from build123d import *

# Parameters (mm, degrees)
BOSS_EXTRUDE1_DEPTH      = 25
CUT_EXTRUDE1_DEPTH       = 4
FILLET1_R                = 4
FILLET2_R                = 10
FILLET3_R                = 5
FILLET4_R                = 3
BOSS_EXTRUDE2_DEPTH      = 3
BOSS_EXTRUDE2_DEPTH_BACK = 3
FILLET5_R                = 3


with BuildPart() as part:
    # Sketch1 → Boss-Extrude1 (new body)
    with BuildSketch(Plane(origin=(0, 0, 0), x_dir=(0, 0, -1), z_dir=(1, 0, 0))):
        Polygon((0, 0), (-130, 0), (-130, 5), (-100.000366453, 5.148280317), (-77.868517379, 27.5), (101.088229162, 27.5), (114, 18), (114, 0), (74, 0), (74, 7.5), (0, 7.5), align=None)
    extrude(amount=BOSS_EXTRUDE1_DEPTH)

    # Sketch4 → Cut-Extrude1 (cut)
    with BuildSketch(Plane(origin=(25, 0, 0), x_dir=(0, 0, -1), z_dir=(1, 0, 0))):
        Polygon((-100.876178749, 0), (0, 0), (111, 0), (111, 3), (111, 16.482758557), (100.103496394, 24.5), (-76.617181678, 24.5), align=None)
    cut_extrude1 = extrude(amount=-CUT_EXTRUDE1_DEPTH, mode=Mode.SUBTRACT)

    # Mirror2: Cut-Extrude1 across plane
    add(cut_extrude1.mirror(Plane(origin=(12.5, 0, 0), x_dir=(0, 0, 1), z_dir=(1, 0, 0))), mode=Mode.SUBTRACT)

    # Fillet1
    fillet1_edges = [part.edges().sort_by_distance(p)[0] for p in [
        (12.5, 7.5, -74),
        (12.5, 7.5, 0),
    ]]
    fillet(fillet1_edges, radius=FILLET1_R)

    # Fillet2
    fillet2_edges = [part.edges().sort_by_distance(p)[0] for p in [
        (23, 0, 100.876178749),
        (23, 24.5, 76.617181678),
        (23, 24.5, -100.103496394),
        (23, 16.482758557, -111),
        (2, 0, 100.876178749),
        (2, 16.482758557, -111),
        (2, 24.5, -100.103496394),
        (2, 24.5, 76.617181678),
    ]]
    fillet(fillet2_edges, radius=FILLET2_R)

    # Fillet3
    fillet3_edges = [part.edges().sort_by_distance(p)[0] for p in [
        (12.5, 5.148280317, 100.000366453),
        (12.5, 27.5, 77.868517379),
        (12.5, 27.5, -101.088229162),
        (12.5, 18, -114),
    ]]
    fillet(fillet3_edges, radius=FILLET3_R)

    # Fillet4
    fillet4_edges = [part.edges().sort_by_distance(p)[0] for p in [
        (0, 2.5, 130),
        (25, 2.5, 130),
    ]]
    fillet(fillet4_edges, radius=FILLET4_R)

    # Sketch5 → Boss-Extrude2 (add, two sides: drawn at the far end of the back side and taken through both)
    with BuildSketch(Plane(origin=(12.5, 0, 0), x_dir=(0, 0, -1), z_dir=(1, 0, 0)).offset(-BOSS_EXTRUDE2_DEPTH_BACK)):
        Polygon((-117.8659777, 5.059975288), (-103.793914836, 19.271838176), (-72.605250228, 19.271838176), (-95.8659777, 5.059975288), align=None)
    extrude(amount=BOSS_EXTRUDE2_DEPTH + BOSS_EXTRUDE2_DEPTH_BACK)

    # Fillet5
    fillet5_edges = [part.edges().sort_by_distance(p)[0] for p in [
        (12.5, 19.271838176, 103.793914836),
    ]]
    fillet(fillet5_edges, radius=FILLET5_R)


solid = part.part
Read the model definition and answer for the solid it produces. Units are mm, in the model's axes. A direction names the side the tool comes from. Coordinates: 2 decimals unless noted, no trailing zeros. Write each loop counter-clockwise with the first axis right and the second up, starting at its lowest first coordinate (ties: lowest second). Pieces come first, ordered by that corner, then holes. Notation, with made-up numbers: (-23, -28.75) -> (6, -28.75) arc R25 ccw to (6, -3.75) -> close; hole circle Ø9 at (-32.5, -30). An arc over 180 degrees is marked (long way). Return JSON: item names as keys, results as strings.
(1) Consider line 1 along Z through (x, y) = (11.5, 2.25); line 2 along X through (y, z) = (11, -64); line 3 along Y through (x, z) = (22, 56). Determine where each line is inside the solid, lowest interval first. Write a range as from..to.
Answers below:
{"line 1": "-114..-74, 0..130", "line 2": "4..21", "line 3": "24.5..27.5"}
(2) The part is cut by section C-C on z = -83.5. Give the vertices of the cut face in (x, y).
Answers below:
{"outline": "(0, 24.5) -> (4, 24.5) -> (4, 0) -> (21, 0) -> (21, 24.5) -> (25, 24.5) -> (25, 27.5) -> (0, 27.5) -> close"}
(3) Each of these flat-tipped pins is pushed along its axis until it touches: P1, Ø2, axis at y = 20, z = -54.5, coming from the -X side; P2, Ø3, axis at y = 14.5, z = -80, coming from the +X side; P3, Ø2, axis at x = 22.5, z = 95, coming from the -Y side; P4, Ø7, axis at y = 9.5, z = 94.5, coming from the -X side. Where does it stop, or does it pass through?
Answers below:
{"P1": "x = 4", "P2": "x = 21", "P3": "y = 4.92", "P4": "x = 0"}
(4) The part is cut by section B-B on x = 7.25. Give the vertices of the cut face in (y, z), then the cut area to 3 significant figures.
Answers below:
{"outline": "(0, -114) -> (15.47, -114) arc R5 ccw to (19.5, -111.96) -> (26.53, -102.41) arc R5 ccw to (27.5, -99.45) -> (27.5, 75.78) arc R5 ccw to (26.02, 79.34) -> (6.62, 98.54) arc R5 cw to (5.14, 102.07) -> (5, 130) -> (0, 130) -> (0, 0) -> (3.5, 0) arc R4 cw to (7.5, -4) -> (7.5, -70) arc R4 cw to (3.5, -74) -> (0, -74) -> close", "area": "5,180 mm^2"}
(5) The part is cut by section A-A on z = -45. Give the vertices of the cut face in (x, y).
Answers below:
{"outline": "(0, 24.5) -> (4, 24.5) -> (4, 7.5) -> (21, 7.5) -> (21, 24.5) -> (25, 24.5) -> (25, 27.5) -> (0, 27.5) -> close"}
(6) Which of the six approach directions +Z, -Z, +X, -X, +Y, -Y give full straight-line access (tool end or side, diameter ignored) to faces 5 (the flat face through (9.5, 12, 102)), 6 (the cylindrical face through (2.03, 0.75, 101.25)), 7 (the flat face through (21, 12, -1))?
Answers below:
{"face 5": "+Z, -X, +Y", "face 6": "-X, -Y", "face 7": "+X, -Y"}
(7) For a pull along Z with two mould halves and no side action, classify faces 1 (the cylindrical face through (22.972, 15.88, -109.953)), 2 (the flat face through (12.32, 23.06, -107.12)), 3 (the flat face through (12, 0, -94)), 4 (the flat face through (1.972, 20.996, -104.866)) as pulls with the +Z half, pulls with the -Z half, needs draft (parallel to the pull), parting line crosses it, or undercut.
Answers below:
{"face 1": "undercut", "face 2": "pulls with the -Z half", "face 3": "needs draft", "face 4": "undercut"}
